from build123d import *

# Parameters (mm, degrees)
SKETCH_1_W          = 20
SKETCH_1_H          = 38
EXTRUDE_1_DEPTH     = 3
SKETCH_2_W          = 20
SKETCH_2_H          = 3
EXTRUDE_2_DEPTH     = 35
SKETCH_3_R          = 2.5
CUT_EXTRUDE_1_DEPTH = 10
SKETCH_4_R          = 1.5
CUT_EXTRUDE_2_DEPTH = 10


with BuildPart() as part:
    # 草图1 → 凸台-拉伸1 (new body)
    with BuildSketch(Plane.XY):
        Rectangle(SKETCH_1_W, SKETCH_1_H)
    extrude(amount=EXTRUDE_1_DEPTH)

    # 草图2 → 凸台-拉伸2 (add)
    with BuildSketch(Plane.XY.offset(3)):
        with Locations((0, -17.5)):
            Rectangle(SKETCH_2_W, SKETCH_2_H)
    extrude(amount=EXTRUDE_2_DEPTH)

    # 草图3 → 切除-拉伸1 (cut)
    with BuildSketch(Plane(origin=(0, 0, 0), x_dir=(-1, 0, 0), z_dir=(0, 0, -1))):
        with Locations((0, 5.915992135)):
            Circle(SKETCH_3_R)
    extrude(amount=-CUT_EXTRUDE_1_DEPTH, mode=Mode.SUBTRACT)

    # 草图4 → 切除-拉伸2 (cut)
    with BuildSketch(Plane(origin=(0, -16, 0), x_dir=(1, 0, 0), z_dir=(0, 1, 0))):
        with Locations(Location((-5, -13, 0), (0, 0, 270))):
            Circle(SKETCH_4_R)
        with Locations(Location((5, -13, 0), (0, 0, 270))):
            Circle(SKETCH_4_R)
    extrude(amount=-CUT_EXTRUDE_2_DEPTH, mode=Mode.SUBTRACT)


solid = part.part
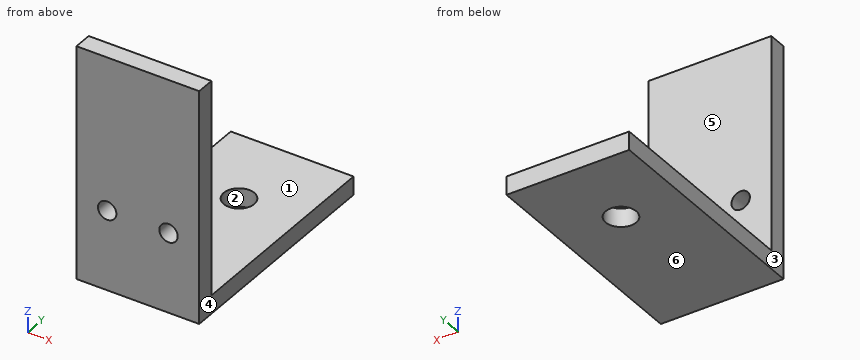
Verification items for the finished model (mm, model axes). Face numbers are marked on the shaded views. A direction names the side the tool comes from. Coordinates: 2 decimals unless noted, no trailing zeros. Write each loop counter-clockwise with the first axis right and the second up, starting at its lowest first coordinate (ties: lowest second). Pieces come first, ordered by that corner, then holes. Notation, with made-up numbers: M -18.5,87.25 L 12.5,87.25 A31 ccw 12.5,124.25 Z; hole C 1.25,4.5 d8. An arc over 180 degrees is marked long. Use CSV: the item, a comma, the result in double quotes.
Q1. Mould release check, pull along X, two halves, no side actions. Record for the marked faces 1, 2, 3 and 4: pulls with the +X half, pulls with the -X half, needs draft (parallel to the pull), parting line crosses it, or undercut.
Computed values:
face 1,"needs draft"
face 2,"undercut"
face 3,"pulls with the -X half"
face 4,"pulls with the +X half"
Q2. Set-up check for the marked faces 5 and 6: record each of +Z, -Z, +X, -X, +Y, -Y from which the full face is reachable in a straight line by a thin tool's end or side.
Computed values:
face 5,"+Z, +X, -X, +Y"
face 6,"-Z, +X, -X, +Y, -Y"
Q3. Section check C-C, the plane x = -9. Enter the section's corners in (y, z).
Computed values:
outline,"M -19,0 L 19,0 L 19,3 L -16,3 L -16,38 L -19,38 Z"
Q4. Section check D-D, the plane x = 0. Enter the section's corners in (y, z), and give its area (3 significant figures).
Computed values:
outline,"M -19,0 L 3.42,0 L 3.42,3 L -16,3 L -16,38 L -19,38 Z; M 8.42,0 L 19,0 L 19,3 L 8.42,3 Z"
area,"204 mm²"
Q5. Go/stop test with flat-tipped pins: P1, Ø1, axis at x = 4, z = 24.5, coming from the +Y side; P2, Ø6, axis at x = -1.5, y = -6.5, coming from the -Z side; P3, Ø3, axis at x = -1.5, y = -4.5, coming from the +Z side. Record where each tip stops, or that it passes through.
Computed values:
P1,"y = -16"
P2,"z = 0"
P3,"z = 3"
Q6. Section check A-A, the plane z = 13. Enter the section's corners in (x, y), and give its area (3 significant figures).
Computed values:
outline,"M -10,-19 L -6.5,-19 L -6.5,-16 L -10,-16 Z; M -3.5,-19 L 3.5,-19 L 3.5,-16 L -3.5,-16 Z; M 6.5,-19 L 10,-19 L 10,-16 L 6.5,-16 Z"
area,"42.0 mm²"
Q7. Thickness scan on line 1 along X through (y, z) = (-18.1, 13); line 2 along Z through (x, y) = (-4.25, -7); line 3 along Y through (x, z) = (4.5, 29). Record the ranges inside material, lowest first. Write a range as [from, to].
Computed values:
line 1,"[-10, -6.5], [-3.5, 3.5], [6.5, 10]"
line 2,"[0, 3]"
line 3,"[-19, -16]"
Q8. Section check B-B, the plane x = -5. Enter the section's corners in (y, z).
Computed values:
outline,"M -19,0 L 19,0 L 19,3 L -16,3 L -16,11.5 L -19,11.5 Z; M -19,14.5 L -16,14.5 L -16,38 L -19,38 Z"
